For this review, take the finished solid that the model builds, in its own axes (mm). A direction names the side the tool comes from. Give positions to 0.01 mm unless a question says otherwise; leave off trailing zeros. Loops run counter-clockwise (first coordinate to the right, second up) from the corner with the lowest first, then second, coordinate; pieces in that order, holes last.
```python
from build123d import *

# Parameters (mm, degrees)
BOSS_EXTRU_1_DEPTH                   = 6
ENL_V_MAT_EXTRU_10_REACH             = 214.217
ESQUISSE12_R                         = 7.5
SYM_TRIE10_COPY_1_REACH              = 214.217
SYM_TRIE10_COPY_1_SKETCH_R           = 7.5
ENL_V_MAT_EXTRU_11_REACH             = 214.217
ESQUISSE13_R                         = 4.3
ESQUISSE13_R_2                       = 1.5
ENL_V_MAT_EXTRU_12_REACH             = 214.217
CONG_1_R                             = 4
CONG_1_OF_SYM_TRIE11_R               = 4
ENL_V_MAT_EXTRU_13_REACH             = 214.217
ESQUISSE15_R                         = 2.3
ENL_V_MAT_EXTRU_13_DIRECTION_2_DEPTH = 213.216870206
R_P_TITION_LIN_AIRE1_COUNT           = 2
R_P_TITION_LIN_AIRE1_PITCH           = 105
ENL_V_MAT_EXTRU_14_DEPTH             = 24
ENL_V_MAT_EXTRU_15_REACH             = 202.908
ESQUISSE17_W                         = 25
ESQUISSE17_H                         = 45
CONG_2_R                             = 6


with BuildPart() as part:
    # Esquisse1 → Boss.-Extru.1 (new body)
    with BuildSketch(Plane(origin=(0, 0, 0), x_dir=(1, 0, 0), z_dir=(0, 1, 0))):
        Polygon((-150, 0), (-150, 120), (-120, 150), (0, 150), (120, 150), (150, 120), (150, 0), (150, -120), (120, -150), (0, -150), (-120, -150), (-150, -120), align=None)
    extrude(amount=BOSS_EXTRU_1_DEPTH)

    # Esquisse12 → Enl_v. mat.-Extru.10 (cut, up to next)
    with BuildSketch(Plane(origin=(0, 6, 0), x_dir=(1, 0, 0), z_dir=(0, 1, 0)), mode=Mode.PRIVATE) as enl_v_mat_extru_10_sk1:
        with Locations(Location((-114.854021031, 97.087596514, 0), (0, 0, 270))):
            Circle(ESQUISSE12_R)
    enl_v_mat_extru_10_tool1 = extrude(enl_v_mat_extru_10_sk1.sketch, amount=-ENL_V_MAT_EXTRU_10_REACH, mode=Mode.PRIVATE) & part.part
    enl_v_mat_extru_10 = enl_v_mat_extru_10_tool1.solids().sort_by_distance((-114.854021, 6, -97.087597))[0]
    add(enl_v_mat_extru_10, mode=Mode.SUBTRACT)

    # Sym_trie9: Enl_v. mat.-Extru.10 across plane
    add(enl_v_mat_extru_10.mirror(Plane(origin=(0, 0, 0), x_dir=(0, 0, 1), z_dir=(1, 0, 0))), mode=Mode.SUBTRACT)

    # Sym_trie10: Enl_v. mat.-Extru.10 across plane
    add(enl_v_mat_extru_10.mirror(Plane.XY), mode=Mode.SUBTRACT)

    # Sym_trie10 copy 1 sketch → Sym_trie10 copy 1 (cut, up to next)
    with BuildSketch(Plane(origin=(0, 6, 0), x_dir=(-1, 0, 0), z_dir=(0, 1, 0)), mode=Mode.PRIVATE) as sym_trie10_copy_1_sk1:
        with Locations(Location((-114.854021031, 97.087596514, 0), (0, 0, 270))):
            Circle(SYM_TRIE10_COPY_1_SKETCH_R)
    sym_trie10_copy_1_tool1 = extrude(sym_trie10_copy_1_sk1.sketch, amount=-SYM_TRIE10_COPY_1_REACH, mode=Mode.PRIVATE) & part.part
    add(sym_trie10_copy_1_tool1.solids().sort_by_distance((114.854021, 6, 97.087597))[0], mode=Mode.SUBTRACT)

    # Esquisse13 → Enl_v. mat.-Extru.11 (cut, up to next)
    with BuildSketch(Plane(origin=(0, 6, 0), x_dir=(1, 0, 0), z_dir=(0, 1, 0)), mode=Mode.PRIVATE) as enl_v_mat_extru_11_sk1:
        with Locations(Location((0, 0, 0), (0, 0, 270))):
            Circle(ESQUISSE13_R)
    enl_v_mat_extru_11_tool1 = extrude(enl_v_mat_extru_11_sk1.sketch, amount=-ENL_V_MAT_EXTRU_11_REACH, mode=Mode.PRIVATE) & part.part
    # Esquisse13 → Enl_v. mat.-Extru.11 (cut, up to next)
    with BuildSketch(Plane(origin=(0, 6, 0), x_dir=(1, 0, 0), z_dir=(0, 1, 0)), mode=Mode.PRIVATE) as enl_v_mat_extru_11_sk2:
        with Locations(Location((8, 0, 0), (0, 0, 270))):
            Circle(ESQUISSE13_R_2)
    enl_v_mat_extru_11_tool2 = extrude(enl_v_mat_extru_11_sk2.sketch, amount=-ENL_V_MAT_EXTRU_11_REACH, mode=Mode.PRIVATE) & part.part
    # Esquisse13 → Enl_v. mat.-Extru.11 (cut, up to next)
    with BuildSketch(Plane(origin=(0, 6, 0), x_dir=(1, 0, 0), z_dir=(0, 1, 0)), mode=Mode.PRIVATE) as enl_v_mat_extru_11_sk3:
        with Locations(Location((0, -8, 0), (0, 0, 270))):
            Circle(ESQUISSE13_R_2)
    enl_v_mat_extru_11_tool3 = extrude(enl_v_mat_extru_11_sk3.sketch, amount=-ENL_V_MAT_EXTRU_11_REACH, mode=Mode.PRIVATE) & part.part
    # Esquisse13 → Enl_v. mat.-Extru.11 (cut, up to next)
    with BuildSketch(Plane(origin=(0, 6, 0), x_dir=(1, 0, 0), z_dir=(0, 1, 0)), mode=Mode.PRIVATE) as enl_v_mat_extru_11_sk4:
        with Locations(Location((0, 8, 0), (0, 0, 270))):
            Circle(ESQUISSE13_R_2)
    enl_v_mat_extru_11_tool4 = extrude(enl_v_mat_extru_11_sk4.sketch, amount=-ENL_V_MAT_EXTRU_11_REACH, mode=Mode.PRIVATE) & part.part
    # Esquisse13 → Enl_v. mat.-Extru.11 (cut, up to next)
    with BuildSketch(Plane(origin=(0, 6, 0), x_dir=(1, 0, 0), z_dir=(0, 1, 0)), mode=Mode.PRIVATE) as enl_v_mat_extru_11_sk5:
        with Locations(Location((-8, 0, 0), (0, 0, 270))):
            Circle(ESQUISSE13_R_2)
    enl_v_mat_extru_11_tool5 = extrude(enl_v_mat_extru_11_sk5.sketch, amount=-ENL_V_MAT_EXTRU_11_REACH, mode=Mode.PRIVATE) & part.part
    add(enl_v_mat_extru_11_tool1.solids().sort_by_distance((0, 6, 0))[0], mode=Mode.SUBTRACT)
    add(enl_v_mat_extru_11_tool2.solids().sort_by_distance((8, 6, 0))[0], mode=Mode.SUBTRACT)
    add(enl_v_mat_extru_11_tool3.solids().sort_by_distance((0, 6, 8))[0], mode=Mode.SUBTRACT)
    add(enl_v_mat_extru_11_tool4.solids().sort_by_distance((0, 6, -8))[0], mode=Mode.SUBTRACT)
    add(enl_v_mat_extru_11_tool5.solids().sort_by_distance((-8, 6, 0))[0], mode=Mode.SUBTRACT)

    # Esquisse14 → Enl_v. mat.-Extru.12 (cut, up to next)
    with BuildSketch(Plane(origin=(0, 6, 0), x_dir=(1, 0, 0), z_dir=(0, 1, 0)), mode=Mode.PRIVATE) as enl_v_mat_extru_12_sk1:
        Polygon((52.5, -125), (82.5, -125), (82.5, 125), (22.5, 125), (22.5, -125), align=None)
    enl_v_mat_extru_12_tool1 = extrude(enl_v_mat_extru_12_sk1.sketch, amount=-ENL_V_MAT_EXTRU_12_REACH, mode=Mode.PRIVATE) & part.part
    enl_v_mat_extru_12 = enl_v_mat_extru_12_tool1.solids().sort_by_distance((52.5, 6, 0))[0]
    add(enl_v_mat_extru_12, mode=Mode.SUBTRACT)

    # Cong_1
    cong_1_edges = [part.edges().sort_by_distance(p)[0] for p in [
        (22.5, 3, -125),
        (82.5, 3, -125),
        (82.5, 3, 125),
        (22.5, 3, 125),
    ]]
    fillet(cong_1_edges, radius=CONG_1_R)

    # Sym_trie11: Enl_v. mat.-Extru.12 across plane
    add(enl_v_mat_extru_12.mirror(Plane(origin=(0, 0, 0), x_dir=(0, 0, 1), z_dir=(1, 0, 0))), mode=Mode.SUBTRACT)

    # Cong_1 of Sym_trie11
    cong_1_of_sym_trie11_edges = [part.edges().sort_by_distance(p)[0] for p in [
        (-22.5, 3, -125),
        (-82.5, 3, -125),
        (-82.5, 3, 125),
        (-22.5, 3, 125),
    ]]
    fillet(cong_1_of_sym_trie11_edges, radius=CONG_1_OF_SYM_TRIE11_R)

    # Esquisse15 → Enl_v. mat.-Extru.13 (cut, up to next)
    with BuildSketch(Plane(origin=(0, 6, 0), x_dir=(1, 0, 0), z_dir=(0, 1, 0)), mode=Mode.PRIVATE) as enl_v_mat_extru_13_sk1:
        with Locations(Location((-40, 130, 0), (0, 0, 90))):
            Circle(ESQUISSE15_R)
    enl_v_mat_extru_13_tool1 = extrude(enl_v_mat_extru_13_sk1.sketch, amount=-ENL_V_MAT_EXTRU_13_REACH, mode=Mode.PRIVATE) & part.part
    # Esquisse15 → Enl_v. mat.-Extru.13 (cut, up to next)
    with BuildSketch(Plane(origin=(0, 6, 0), x_dir=(1, 0, 0), z_dir=(0, 1, 0)), mode=Mode.PRIVATE) as enl_v_mat_extru_13_sk2:
        with Locations(Location((-40, -130, 0), (0, 0, 90))):
            Circle(ESQUISSE15_R)
    enl_v_mat_extru_13_tool2 = extrude(enl_v_mat_extru_13_sk2.sketch, amount=-ENL_V_MAT_EXTRU_13_REACH, mode=Mode.PRIVATE) & part.part
    enl_v_mat_extru_13_1 = enl_v_mat_extru_13_tool1.solids().sort_by_distance((-40, 6, -130))[0]
    add(enl_v_mat_extru_13_1, mode=Mode.SUBTRACT)
    enl_v_mat_extru_13_2 = enl_v_mat_extru_13_tool2.solids().sort_by_distance((-40, 6, 130))[0]
    add(enl_v_mat_extru_13_2, mode=Mode.SUBTRACT)
    enl_v_mat_extru_13 = enl_v_mat_extru_13_1 + enl_v_mat_extru_13_2  # Enl_v. mat.-Extru.13 as one shape, for the pattern or mirror that repeats it

    # Esquisse15 → Enl_v. mat.-Extru.13 direction 2 (cut)
    with BuildSketch(Plane(origin=(0, 6, 0), x_dir=(1, 0, 0), z_dir=(0, 1, 0))):
        with Locations(Location((-40, 130, 0), (0, 0, 90))):
            Circle(ESQUISSE15_R)
        with Locations(Location((-40, -130, 0), (0, 0, 90))):
            Circle(ESQUISSE15_R)
    enl_v_mat_extru_13_direction_2 = extrude(amount=ENL_V_MAT_EXTRU_13_DIRECTION_2_DEPTH, mode=Mode.SUBTRACT)

    # R_p_tition lin_aire1: Enl_v. mat.-Extru.13, Enl_v. mat.-Extru.13 direction 2 ×2
    with Locations(*[(i * R_P_TITION_LIN_AIRE1_PITCH, 0, 0) for i in range(1, R_P_TITION_LIN_AIRE1_COUNT)]):
        add(enl_v_mat_extru_13, mode=Mode.SUBTRACT)
        add(enl_v_mat_extru_13_direction_2, mode=Mode.SUBTRACT)

    # Esquisse16 → Enl_v. mat.-Extru.14 (cut)
    with BuildSketch(Plane(origin=(0, 6, 0), x_dir=(1, 0, 0), z_dir=(0, 1, 0))):
        Polygon((150, 120), (120, 150), (-120, 150), (-150, 120), (-150, -120), (-120, -150), (120, -150), (150, -120), align=None)
        Polygon((-142, 116.686291501), (-116.686291501, 142), (116.686291501, 142), (142, 116.686291501), (142, -116.686291501), (116.686291501, -142), (-116.686291501, -142), (-142, -116.686291501), align=None, mode=Mode.SUBTRACT)
    extrude(amount=-ENL_V_MAT_EXTRU_14_DEPTH, mode=Mode.SUBTRACT)

    # Esquisse17 → Enl_v. mat.-Extru.15 (cut, up to next)
    with BuildSketch(Plane(origin=(0, 6, 0), x_dir=(1, 0, 0), z_dir=(0, 1, 0)), mode=Mode.PRIVATE) as enl_v_mat_extru_15_sk1:
        Polygon((-117, -45), (-142, -45), (-142, -60), align=None)
    enl_v_mat_extru_15_tool1 = extrude(enl_v_mat_extru_15_sk1.sketch, amount=-ENL_V_MAT_EXTRU_15_REACH, mode=Mode.PRIVATE) & part.part
    # Esquisse17 → Enl_v. mat.-Extru.15 (cut, up to next)
    with BuildSketch(Plane(origin=(0, 6, 0), x_dir=(1, 0, 0), z_dir=(0, 1, 0)), mode=Mode.PRIVATE) as enl_v_mat_extru_15_sk2:
        with Locations((-129.5, -22.5)):
            Rectangle(ESQUISSE17_W, ESQUISSE17_H)
    enl_v_mat_extru_15_tool2 = extrude(enl_v_mat_extru_15_sk2.sketch, amount=-ENL_V_MAT_EXTRU_15_REACH, mode=Mode.PRIVATE) & part.part
    # Esquisse17 → Enl_v. mat.-Extru.15 (cut, up to next)
    with BuildSketch(Plane(origin=(0, 6, 0), x_dir=(1, 0, 0), z_dir=(0, 1, 0)), mode=Mode.PRIVATE) as enl_v_mat_extru_15_sk3:
        with Locations((-129.5, 22.5)):
            Rectangle(ESQUISSE17_W, ESQUISSE17_H)
    enl_v_mat_extru_15_tool3 = extrude(enl_v_mat_extru_15_sk3.sketch, amount=-ENL_V_MAT_EXTRU_15_REACH, mode=Mode.PRIVATE) & part.part
    # Esquisse17 → Enl_v. mat.-Extru.15 (cut, up to next)
    with BuildSketch(Plane(origin=(0, 6, 0), x_dir=(1, 0, 0), z_dir=(0, 1, 0)), mode=Mode.PRIVATE) as enl_v_mat_extru_15_sk4:
        Polygon((-142, 60), (-142, 45), (-117, 45), align=None)
    enl_v_mat_extru_15_tool4 = extrude(enl_v_mat_extru_15_sk4.sketch, amount=-ENL_V_MAT_EXTRU_15_REACH, mode=Mode.PRIVATE) & part.part
    enl_v_mat_extru_15_1 = enl_v_mat_extru_15_tool1.solids().sort_by_distance((-133.666667, 6, 50))[0]
    add(enl_v_mat_extru_15_1, mode=Mode.SUBTRACT)
    enl_v_mat_extru_15_2 = enl_v_mat_extru_15_tool2.solids().sort_by_distance((-129.5, 6, 22.5))[0]
    add(enl_v_mat_extru_15_2, mode=Mode.SUBTRACT)
    enl_v_mat_extru_15_3 = enl_v_mat_extru_15_tool3.solids().sort_by_distance((-129.5, 6, -22.5))[0]
    add(enl_v_mat_extru_15_3, mode=Mode.SUBTRACT)
    enl_v_mat_extru_15_4 = enl_v_mat_extru_15_tool4.solids().sort_by_distance((-133.666667, 6, -50))[0]
    add(enl_v_mat_extru_15_4, mode=Mode.SUBTRACT)
    enl_v_mat_extru_15 = enl_v_mat_extru_15_1 + enl_v_mat_extru_15_2 + enl_v_mat_extru_15_3 + enl_v_mat_extru_15_4  # Enl_v. mat.-Extru.15 as one shape, for the pattern or mirror that repeats it

    # Sym_trie12: Enl_v. mat.-Extru.15 across plane
    add(enl_v_mat_extru_15.mirror(Plane(origin=(0, 0, 0), x_dir=(0, 0, 1), z_dir=(1, 0, 0))), mode=Mode.SUBTRACT)

    # Cong_2
    cong_2_edges = [part.edges().sort_by_distance(p)[0] for p in [
        (116.686291501, 3, -142),
        (-116.686291501, 3, -142),
        (-142, 3, -116.686291501),
        (-142, 3, 116.686291501),
        (-116.686291501, 3, 142),
        (116.686291501, 3, 142),
        (142, 3, 116.686291501),
        (142, 3, -116.686291501),
        (-117, 3, 45),
        (-142, 3, 60),
        (-142, 3, -60),
        (-117, 3, -45),
        (142, 3, 60),
        (117, 3, 45),
        (117, 3, -45),
        (142, 3, -60),
    ]]
    fillet(cong_2_edges, radius=CONG_2_R)


solid = part.part
```
Q1. Consider section A-A on x = 47.5. Give the boundary of the cut face in (y, z).
Answers:
outline: (0, -142) - (6, -142) - (6, -125) - (0, -125) - close; (0, 125) - (6, 125) - (6, 142) - (0, 142) - close
Q2. For probe 1 along X at (y, z) = (5.25, -31); probe 2 along X at (y, z) = (1.3, 0); probe 3 along X at (y, z) = (3, -107.5), list the stretches that pass through material, from the lowest coordinate up.
Answers:
probe 1: x = -117 to -82.5, -22.5 to 22.5, 82.5 to 117
probe 2: x = -117 to -82.5, -22.5 to -9.5, -6.5 to -4.3, 4.3 to 6.5, 9.5 to 22.5, 82.5 to 117
probe 3: x = -142 to -82.5, -22.5 to 22.5, 82.5 to 142
Q3. Consider section B-B on z = 93. Give the boundary of the cut face in (x, y).
Answers:
outline: (-142, 0) - (-121.14, 0) - (-121.14, 6) - (-142, 6) - close; (-108.57, 0) - (-82.5, 0) - (-82.5, 6) - (-108.57, 6) - close; (-22.5, 0) - (22.5, 0) - (22.5, 6) - (-22.5, 6) - close; (82.5, 0) - (108.57, 0) - (108.57, 6) - (82.5, 6) - close; (121.14, 0) - (142, 0) - (142, 6) - (121.14, 6) - close
Q4. For pin 1 Ø3 at (y, z) = (4.5, 5.5) entering from -X, flat-tipped, find the tip position at first contact; note if it passes through.
Answers:
pin 1: stops at x = -117
Q5. Mouldability with a two-part tool opening along Z and no side actions: class faces 1 (the flat face through (-129.191, 3.042, 129.496)), 2 (the cylindrical face through (114.52, 3.04, -104.58)), 3 (the flat face through (129.191, 3.042, -129.496)) as +Z half, -Z half, draft (parallel to the pull), parting line (faces both ways), or undercut.
Answers:
face 1: +Z half
face 2: undercut
face 3: -Z half
Q6. Machinability: for faces 4 (the cylindrical face through (-2.62, 3.04, -3.41)), 5 (the flat face through (129.37, 3.04, -52.42)), 6 (the flat face through (-129.63, 3.04, 52.58)), which of the approach directions +Z, -Z, +X, -X, +Y, -Y give a long, thin tool a straight path to every point of the face, cutting with its end or side? Answer none if there is none.
Answers:
face 4: +Y, -Y
face 5: +X, +Y, -Y
face 6: -X, +Y, -Y
Q7. Consider section C-C on y = 2. Count the separate pieces of the cut face and the enclosed holes in it, plus the area to 3 significant figures.
Answers:
separate pieces: 1
enclosed holes: 15
area: 43,300 mm2
